Part print with two shaded views. Sizes in mm from the minimum x, y, z corner. A direction names the side the tool comes from. Coordinates: 2 decimals unless noted, no trailing zeros. Write each loop counter-clockwise with the first axis right and the second up, starting at its lowest first coordinate (ties: lowest second). Pieces come first, ordered by that corner, then holes. Notation, with made-up numbers: M 78.5,49.25 L 105.5,49.25 A8 cw 105.5,53.25 Z; hole C -32,-16 d5. An arc over 180 degrees is marked long. Use CSV: the item, a comma, the result in double quotes. Start each with the question number.
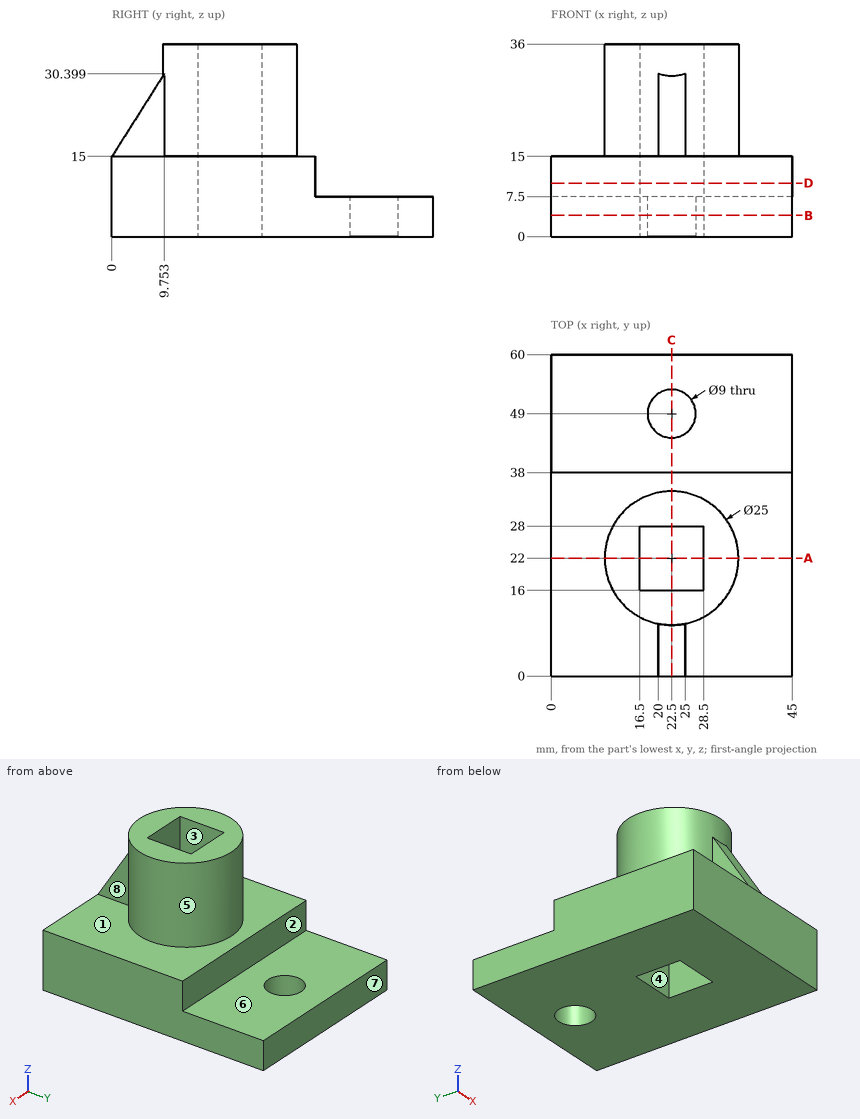
1. Flat gauge pins, fed straight in: pin 1 (6 mm diameter, centred on x = 28, y = 43, fed in from -Z); pin 2 (6 mm diameter, centred on x = 5.5, y = 52, fed in from +Z); pin 3 (9.5 mm diameter, centred on y = 23, z = 21, fed in from +X); pin 4 (8 mm diameter, centred on y = 3.5, z = 23, fed in from +X). Where does each tip first touch, or does it go through?
2. Slice it at C-C (x = 22.5). List the corners of the cut face in (y, z), and give its area (3 significant figures).
3. Slice it at A-A (y = 22). List the corners of the cut face in (x, z), and give its area (3 significant figures).
4. Slice it at B-B (z = 4). List the corners of the cut face in (x, y).
5. 3-axis set-ups, long thin cutter, end or side, ignore diameter. For the marked faces 4, 5, 6, 7 and 8: which of +Z, -Z, +X, -X, +Y, -Y reach the whole face in a straight line?
6. Drill centre lines: line 1 along Y through (x, z) = (22.5, 3); line 2 along Y through (x, z) = (18.5, 2) (1 decimal); line 3 along Z through (x, y) = (39, 8.5). Where is each one in solid material? Low to high. Write a range as from..to.
7. Slice it at D-D (z = 10). List the corners of the cut face in (x, y).
8. Pull direction Y, two halves, no side cores. Call the marked faces 1, 2 and 3: pulls with the +Y half, pulls with the -Y half, needs draft (parallel to the pull), parting line crosses it, or undercut.
Established:
1,pin 1,"stops at z = 0"
1,pin 2,"stops at z = 7.5"
1,pin 3,"stops at x = 35"
1,pin 4,"stops at x = 25"
2,outline,"M 0,0 L 16,0 L 16,36 L 9.5,36 L 9.5,30 L 0,15 Z; M 28,0 L 44.5,0 L 44.5,7.5 L 38,7.5 L 38,15 L 34.5,15 L 34.5,36 L 28,36 Z; M 53.5,0 L 60,0 L 60,7.5 L 53.5,7.5 Z"
2,area,"832 mm2"
3,outline,"M 0,0 L 16.5,0 L 16.5,36 L 10,36 L 10,15 L 0,15 Z; M 28.5,0 L 45,0 L 45,15 L 35,15 L 35,36 L 28.5,36 Z"
3,area,"768 mm2"
4,outline,"M 0,0 L 45,0 L 45,60 L 0,60 Z; hole M 16.5,16 L 28.5,16 L 28.5,28 L 16.5,28 Z; hole C 22.5,49 d9"
5,face 4,"+Z, -Z"
5,face 5,"+Z"
5,face 6,"+Z, +X, -X, +Y"
5,face 7,"+Z, -Z, +X, -X, +Y"
5,face 8,"+Z, +X, -Y"
6,line 1,"y = 0..16, 28..44.5, 53.5..60"
6,line 2,"y = 0..16, 28..46.9, 51.1..60"
6,line 3,"z = 0..15"
7,outline,"M 0,0 L 45,0 L 45,38 L 0,38 Z; hole M 16.5,16 L 28.5,16 L 28.5,28 L 16.5,28 Z"
8,face 1,"needs draft"
8,face 2,"pulls with the +Y half"
8,face 3,"undercut"
